from build123d import *

# Parameters (mm, degrees)
SKETCH2_R           = 7.5
BOSS_EXTRUDE1_DEPTH = 1.5
SKETCH3_W           = 25
SKETCH3_H           = 3
CUT_EXTRUDE1_DEPTH  = 4
SKETCH4_W           = 3
SKETCH4_H           = 20
BOSS_EXTRUDE2_DEPTH = 3
SKETCH5_R           = 1.5
CUT_EXTRUDE2_DEPTH  = 10


with BuildPart() as part:
    # Sketch2 → Boss-Extrude1 (new, symmetric)
    with BuildSketch(Plane(origin=(0, 0, 0), x_dir=(0, 0, -1), z_dir=(1, 0, 0))):
        with BuildLine():
            Line((50, 0), (-50, 0))
            Line((-50, 0), (-20, 180))
            ThreePointArc((-20, 180), (0, 200), (20, 180))
            Line((20, 180), (50, 0))
        make_face()
        with Locations((0, 180)):
            Circle(SKETCH2_R, mode=Mode.SUBTRACT)
    extrude(amount=BOSS_EXTRUDE1_DEPTH, both=True)

    # Sketch3 → Cut-Extrude1 (cut)
    with BuildSketch(Plane.ZY.offset(1.5)):
        with Locations((22.5, 34.5)):
            Rectangle(SKETCH3_W, SKETCH3_H)
        with Locations((-22.5, 34.5)):
            Rectangle(SKETCH3_W, SKETCH3_H)
    extrude(amount=-CUT_EXTRUDE1_DEPTH, mode=Mode.SUBTRACT)

    # Sketch4 → Boss-Extrude2 (add)
    with BuildSketch(Plane.XZ):
        Rectangle(SKETCH4_W, SKETCH4_H)
        with Locations((0, -40)):
            Rectangle(SKETCH4_W, SKETCH4_H)
        with Locations((0, 40)):
            Rectangle(SKETCH4_W, SKETCH4_H)
    extrude(amount=BOSS_EXTRUDE2_DEPTH)

    # Sketch5 → Cut-Extrude2 (cut)
    with BuildSketch(Plane(origin=(1.5, 0, 0), x_dir=(0, 0, -1), z_dir=(1, 0, 0))):
        with Locations((-5.5, 193.5)):
            Circle(SKETCH5_R)
        with Locations((-5.5, 164.5)):
            Circle(SKETCH5_R)
        with Locations((5.5, 164.5)):
            Circle(SKETCH5_R)
        with Locations((5.5, 193.5)):
            Circle(SKETCH5_R)
    extrude(amount=-CUT_EXTRUDE2_DEPTH, mode=Mode.SUBTRACT)


solid = part.part
Geometry: final body of the model. Coordinates: model frame, mm. Give positions to 0.01 mm unless a question says otherwise; leave off trailing zeros. Loops run counter-clockwise (first coordinate to the right, second up) from the corner with the lowest first, then second, coordinate; pieces in that order, holes last. Notation, with made-up numbers: (-5.5, -39) -> (30.5, -39) arc R25 cw to (30.5, -5) -> close; hole circle Ø11 at (-3.5, 38.25). An arc over 180 degrees is marked (long way). Put each result on its own line as item: value.
1. Ray query, line 1 along Z through (x, y) = (-0.2, 193.5); line 2 along Z through (x, y) = (0.05, 164.5); line 3 along Y through (x, z) = (0.5, 0). Return the intervals inside material, ascending. Write a range as [from, to].
Taken from the geometry:
line 1: z = [-14.76, -7], [-4, 4], [7, 14.76]
line 2: z = [-22.58, -7], [-4, 4], [7, 22.58]
line 3: y = [-3, 172.5], [187.5, 200]
2. Cut plane C-C (z = 13.5). Return the cut outline in (x, y).
Taken from the geometry:
outline: (-1.5, 0) -> (1.5, 0) -> (1.5, 33) -> (-1.5, 33) -> close; (-1.5, 36) -> (1.5, 36) -> (1.5, 194.76) -> (-1.5, 194.76) -> close
3. Cut plane B-B (x = -0.8). Return the cut outline in (y, z), plus the area to 3 significant figures.
Taken from the geometry:
outline: (-3, -50) -> (0, -50) -> (180, -20) arc R20 ccw to (180, 20) -> (0, 50) -> (-3, 50) -> (-3, 30) -> (0, 30) -> (0, 10) -> (-3, 10) -> (-3, -10) -> (0, -10) -> (0, -30) -> (-3, -30) -> close; hole (33, -35) -> (36, -35) -> (36, -10) -> (33, -10) -> close; hole (33, 10) -> (36, 10) -> (36, 35) -> (33, 35) -> close; hole circle Ø3 at (164.5, -5.5); hole circle Ø3 at (164.5, 5.5); hole circle Ø15 at (180, 0); hole circle Ø3 at (193.5, -5.5); hole circle Ø3 at (193.5, 5.5)
area: 13,100 mm2
4. Pin query (flat end, axial travel): P1, Ø1, axis at x = -1, y = 108, coming from the -Z side; P2, Ø1.5, axis at x = 0.5, z = 17, coming from the -Y side; P3, Ø9, axis at y = 180, z = 0, coming from the -X side (3 decimals); P4, Ø4, axis at y = 164.5, z = 5.5, coming from the +X side. Return the tip coordinate at first contact, or that it passes through.
Taken from the geometry:
P1: stops at z = -32.08
P2: stops at y = 0
P3: passes through
P4: stops at x = 1.5
5. Cut plane D-D (y = 105). Return the cut outline in (x, z).
Taken from the geometry:
outline: (-1.5, -32.5) -> (1.5, -32.5) -> (1.5, 32.5) -> (-1.5, 32.5) -> close
6. Pull-direction query (Z, two-part tool) for faces 1 (the flat face through (1.5, 77, -1)), 2 (the cylindrical face through (0, 200, 0)), 3 (the cylindrical face through (-0.021, 187.436, 0.976)); classes: released by +Z, released by -Z, zero draft, split by the parting line, or undercut.
Taken from the geometry:
face 1: zero draft
face 2: split by the parting line
face 3: undercut
7. Cut plane A-A (z = -16). Return the cut outline in (x, y), plus the area to 3 significant figures.
Taken from the geometry:
outline: (-1.5, 0) -> (1.5, 0) -> (1.5, 33) -> (-1.5, 33) -> close; (-1.5, 36) -> (1.5, 36) -> (1.5, 192) -> (-1.5, 192) -> close
area: 567 mm2
